Verification items for the finished model (mm, model axes). Face numbers are marked on the shaded views. Give positions to 0.01 mm unless a question says otherwise; leave off trailing zeros. Order: outer loops, then holes, each group sorted by start corner. A loop starts at its lowest first (then second) coordinate and runs counter-clockwise, first axis right, second up. Notation, with made-up numbers: (6, 22.5) -> (39, 22.5) arc R23 cw to (39, 35.5) -> close; hole circle Ø5 at (-17, -21). An arc over 180 degrees is marked (long way). One line per question, with ' | ' between items. Start each with the question number.
Q1. Material ranges on probe 1 along Y at (x, z) = (10, 20); probe 2 along X at (y, z) = (-19.5, 3), recorded low to high. Write a range as [from, to].
Q2. Section check A-A on x = 10. Record the cut outline in (y, z).
Q3. Section check B-B on y = -20. Record the cut outline in (x, z), plus the area to 3 significant figures.
Q4. Mould release check, pull along Z, two halves, no side actions. Record for the marked faces 1, 2 and 3: released by +Z, released by -Z, zero draft, split by the parting line, or undercut.
Q5. Section check C-C on z = 22.5. Record the cut outline in (x, y), plus the area to 3 significant figures.
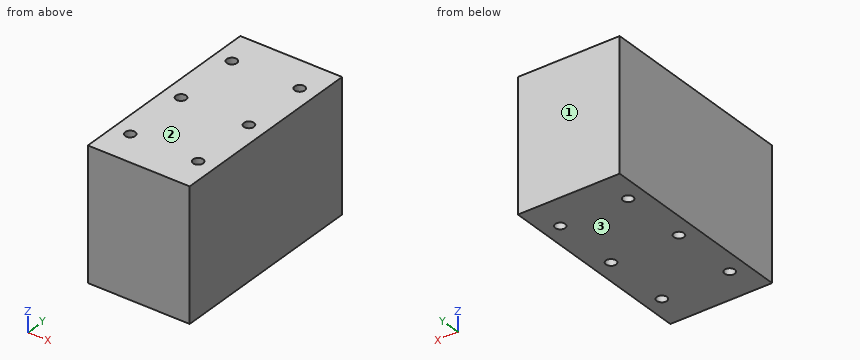
from build123d import *

# Parameters (mm, degrees)
ESQUISSE1_W                     = 30
ESQUISSE1_H                     = 60
EXTRUSION1_DEPTH                = 38.5
ESQUISSE2_R                     = 1.5
EXTRUSION2_DEPTH                = 52.061237744
R_P_TITION_LIN_AIRE1_COUNT      = 3
R_P_TITION_LIN_AIRE1_PITCH      = 20
R_P_TITION_LIN_AIRE1_COUNT_DIR2 = 2
R_P_TITION_LIN_AIRE1_PITCH_DIR2 = 20


with BuildPart() as part:
    # Esquisse1 → Extrusion1 (new body)
    with BuildSketch(Plane.XY):
        Rectangle(ESQUISSE1_W, ESQUISSE1_H)
    extrude(amount=EXTRUSION1_DEPTH)

    # Esquisse2 → Extrusion2 (cut, through all)
    with BuildSketch(Plane.XY.offset(38.5)):
        with Locations((-10, 20)):
            Circle(ESQUISSE2_R)
    extrusion2 = extrude(amount=-EXTRUSION2_DEPTH, mode=Mode.SUBTRACT)

    # Répétition linéaire1: Extrusion2 3 × 2
    with Locations(*[(j * R_P_TITION_LIN_AIRE1_PITCH_DIR2, -i * R_P_TITION_LIN_AIRE1_PITCH, 0) for i in range(R_P_TITION_LIN_AIRE1_COUNT) for j in range(R_P_TITION_LIN_AIRE1_COUNT_DIR2) if (i, j) != (0, 0)]):
        add(extrusion2, mode=Mode.SUBTRACT)


solid = part.part
Filled in:
1) probe 1: [-30, -21.5], [-18.5, -1.5], [1.5, 18.5], [21.5, 30] | probe 2: [-15, -11.41], [-8.59, 8.59], [11.41, 15]
2) outline: (-30, 0) -> (-21.5, 0) -> (-21.5, 38.5) -> (-30, 38.5) -> close; (-18.5, 0) -> (-1.5, 0) -> (-1.5, 38.5) -> (-18.5, 38.5) -> close; (1.5, 0) -> (18.5, 0) -> (18.5, 38.5) -> (1.5, 38.5) -> close; (21.5, 0) -> (30, 0) -> (30, 38.5) -> (21.5, 38.5) -> close
3) outline: (-15, 0) -> (-11.5, 0) -> (-11.5, 38.5) -> (-15, 38.5) -> close; (-8.5, 0) -> (8.5, 0) -> (8.5, 38.5) -> (-8.5, 38.5) -> close; (11.5, 0) -> (15, 0) -> (15, 38.5) -> (11.5, 38.5) -> close | area: 924 mm²
4) face 1: zero draft | face 2: released by +Z | face 3: released by -Z
5) outline: (-15, -30) -> (15, -30) -> (15, 30) -> (-15, 30) -> close; hole circle Ø3 at (-10, -20); hole circle Ø3 at (-10, 0); hole circle Ø3 at (-10, 20); hole circle Ø3 at (10, -20); hole circle Ø3 at (10, 0); hole circle Ø3 at (10, 20) | area: 1,760 mm²
